from build123d import *

# Parameters (mm, degrees)
SKETCH1_R           = 17.5
BOSS_EXTRUDE1_DEPTH = 115


with BuildPart() as part:
    # Sketch1 → Boss-Extrude1 (new body)
    with BuildSketch(Plane(origin=(0, 0, 0), x_dir=(0, 0, -1), z_dir=(1, 0, 0))):
        with BuildLine():
            Line((7.5, 35), (72.5, 35))
            Line((72.5, 35), (72.5, 95))
            Line((72.5, 95), (87.5, 95))
            Line((87.5, 95), (87.5, 35))
            Line((87.5, 35), (152.5, 35))
            Line((152.5, 35), (152.5, 95))
            Line((152.5, 95), (167.5, 95))
            Line((167.5, 95), (167.5, 35))
            Line((167.5, 35), (232.5, 35))
            Line((232.5, 35), (232.5, 95))
            Line((232.5, 95), (247.5, 95))
            Line((247.5, 95), (247.5, 35))
            Line((247.5, 35), (312.5, 35))
            Line((312.5, 35), (312.5, 95))
            Line((312.5, 95), (327.5, 95))
            Line((327.5, 95), (327.5, 35))
            Line((327.5, 35), (392.5, 35))
            Line((392.5, 35), (392.5, 95))
            Line((392.5, 95), (407.5, 95))
            Line((407.5, 95), (407.5, 35))
            Line((407.5, 35), (472.5, 35))
            Line((472.5, 35), (472.5, 95))
            Line((472.5, 95), (487.5, 95))
            Line((487.5, 95), (487.5, 35))
            Line((487.5, 35), (552.5, 35))
            Line((552.5, 35), (552.5, 95))
            Line((552.5, 95), (567.5, 95))
            Line((567.5, 95), (567.5, 35))
            Line((567.5, 35), (632.5, 35))
            Line((632.5, 35), (632.5, 95))
            Line((632.5, 95), (647.5, 95))
            Line((647.5, 95), (647.5, 35))
            Line((647.5, 35), (712.5, 35))
            Line((712.5, 35), (712.5, 95))
            Line((712.5, 95), (727.5, 95))
            Line((727.5, 95), (727.5, 35))
            Line((727.5, 35), (792.5, 35))
            Line((792.5, 35), (792.5, 95))
            Line((792.5, 95), (807.5, 95))
            Line((807.5, 95), (807.5, 34.186985828))
            ThreePointArc((807.5, 34.186985828), (835, 0), (807.5, -34.186985828))
            Line((807.5, -34.186985828), (807.5, -95))
            Line((807.5, -95), (792.5, -95))
            Line((792.5, -95), (792.5, -35))
            Line((792.5, -35), (727.5, -35))
            Line((727.5, -35), (727.5, -95))
            Line((727.5, -95), (712.5, -95))
            Line((712.5, -95), (712.5, -35))
            Line((712.5, -35), (647.5, -35))
            Line((647.5, -35), (647.5, -95))
            Line((647.5, -95), (632.5, -95))
            Line((632.5, -95), (632.5, -35))
            Line((632.5, -35), (567.5, -35))
            Line((567.5, -35), (567.5, -95))
            Line((567.5, -95), (552.5, -95))
            Line((552.5, -95), (552.5, -35))
            Line((552.5, -35), (487.5, -35))
            Line((487.5, -35), (487.5, -95))
            Line((487.5, -95), (472.5, -95))
            Line((472.5, -95), (472.5, -35))
            Line((472.5, -35), (407.5, -35))
            Line((407.5, -35), (407.5, -95))
            Line((407.5, -95), (392.5, -95))
            Line((392.5, -95), (392.5, -35))
            Line((392.5, -35), (327.5, -35))
            Line((327.5, -35), (327.5, -95))
            Line((327.5, -95), (312.5, -95))
            Line((312.5, -95), (312.5, -35))
            Line((312.5, -35), (247.5, -35))
            Line((247.5, -35), (247.5, -95))
            Line((247.5, -95), (232.5, -95))
            Line((232.5, -95), (232.5, -35))
            Line((232.5, -35), (167.5, -35))
            Line((167.5, -35), (167.5, -95))
            Line((167.5, -95), (152.5, -95))
            Line((152.5, -95), (152.5, -35))
            Line((152.5, -35), (87.5, -35))
            Line((87.5, -35), (87.5, -95))
            Line((87.5, -95), (72.5, -95))
            Line((72.5, -95), (72.5, -35))
            Line((72.5, -35), (7.5, -35))
            Line((7.5, -35), (7.5, -95))
            Line((7.5, -95), (-7.5, -95))
            Line((-7.5, -95), (-7.5, -34.186985828))
            ThreePointArc((-7.5, -34.186985828), (-35, 0), (-7.5, 34.186985828))
            Line((-7.5, 34.186985828), (-7.5, 95))
            Line((-7.5, 95), (7.5, 95))
            Line((7.5, 95), (7.5, 35))
        make_face()
        Circle(SKETCH1_R, mode=Mode.SUBTRACT)
        with Locations((800, 0)):
            Circle(SKETCH1_R, mode=Mode.SUBTRACT)
        with Locations((100, 0)):
            Circle(SKETCH1_R, mode=Mode.SUBTRACT)
        with Locations((200, 0)):
            Circle(SKETCH1_R, mode=Mode.SUBTRACT)
        with Locations((300, 0)):
            Circle(SKETCH1_R, mode=Mode.SUBTRACT)
        with Locations((400, 0)):
            Circle(SKETCH1_R, mode=Mode.SUBTRACT)
        with Locations((500, 0)):
            Circle(SKETCH1_R, mode=Mode.SUBTRACT)
        with Locations((600, 0)):
            Circle(SKETCH1_R, mode=Mode.SUBTRACT)
        with Locations((700, 0)):
            Circle(SKETCH1_R, mode=Mode.SUBTRACT)
    extrude(amount=BOSS_EXTRUDE1_DEPTH)


solid = part.part
Model file for the job. Use its own axes, mm. A direction names the side the tool comes from. Round coordinates to 2 decimals unless told otherwise and drop trailing zeros. Order: outer loops, then holes, each group sorted by start corner. A loop starts at its lowest first (then second) coordinate and runs counter-clockwise, first axis right, second up.
(1) Band-saw the part on C-C (z = -600). List the corners of the cut face in (x, y).
(2) Pin check, flat tips, straight feed: pin 1 (18 mm diameter, centred on x = 68.5, y = -66, fed in from -Z); pin 2 (3 mm diameter, centred on x = 29.5, z = -288.5, fed in from -Y); pin 3 (1 mm diameter, centred on x = 31.5, z = -747.5, fed in from +Y); pin 4 (8 mm diameter, centred on x = 73, z = -389, fed in from +Y). Stop position of each tip, or through.
(3) Drill centre lines: line 1 (Y direction, x = 39.5, z = 0); line 2 (Y direction, x = 87.5, z = -499); line 3 (Y direction, x = 104, z = -64). Where is each one in solid material? Low to high.
(4) Band-saw the part on A-A (z = -400). List the corners of the cut face in (x, y).
(5) Band-saw the part on B-B (y = -60). Give the number of separate pieces and of enclosed holes in the cut face, then the cut area to 3 significant figures.
(6) Pull direction Y, two halves, no side cores. Call faces 4 (the face through (56.7, 5.26, -316.69)), 5 (the face through (57, 95, -240)), 6 (the face through (56.7, 5.26, -416.69)), 7 (the face through (57, 65, -152.5)): released by +Y, released by -Y, zero draft, split by the parting line, or undercut.
(7) 3-axis set-ups, long thin cutter, end or side, ignore diameter. For faces 1 (the face through (57, 65, -567.5)), 2 (the face through (57, -35, -200)), 3 (the face through (57, 95, -720)): which of +Z, -Z, +X, -X, +Y, -Y reach the whole face in a straight line?
Verdict:
1. outline: (0, -35) - (115, -35) - (115, -17.5) - (0, -17.5) - close; (0, 17.5) - (115, 17.5) - (115, 35) - (0, 35) - close
2. pin 1: stops at z = -807.5
2. pin 2: stops at y = -35
2. pin 3: stops at y = 35
2. pin 4: stops at y = 95
3. line 1: y = -95 to -17.5, 17.5 to 95
3. line 2: y = -35 to -17.47, 17.47 to 35
3. line 3: y = -35 to 35
4. outline: (0, -95) - (115, -95) - (115, -17.5) - (0, -17.5) - close; (0, 17.5) - (115, 17.5) - (115, 95) - (0, 95) - close
5. separate pieces: 11
5. enclosed holes: 0
5. area: 19,000 mm2
6. face 4: undercut
6. face 5: released by +Y
6. face 6: undercut
6. face 7: zero draft
7. face 1: +X, -X, +Y
7. face 2: +X, -X, -Y
7. face 3: +Z, -Z, +X, -X, +Y
